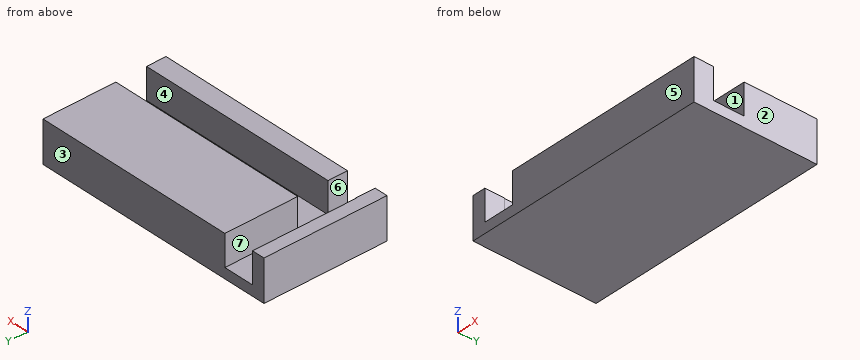
```python
from build123d import *

# Parameters (mm, degrees)
F0_W     = 152.4
F0_H     = 76.2
F1_DEPTH = 25.4
F3_DEPTH = 19.05
F4_W     = 19.05
F4_H     = 19.05
F5_DEPTH = 12.192


with BuildPart() as f1:
    # F0 (on Top) → F1 (new body)
    with BuildSketch(Plane.XY):
        with Locations((24.078096, -6.907338)):
            Rectangle(F0_W, F0_H)
    extrude(amount=F1_DEPTH)

    # F2 (on face) → F3 (cut)
    with BuildSketch(Plane.XY.offset(25.4)):
        Polygon((-25.176978, 31.192662), (-44.226978, 31.192662), (-44.226978, -32.953762), (100.278096, -32.953762), (100.278096, -13.903762), (-25.176978, -13.903762), align=None)
    extrude(amount=-F3_DEPTH, mode=Mode.SUBTRACT)

    # F4 (on face) → F5 (cut)
    with BuildSketch(Plane.XZ.offset(45.007338)):
        with Locations((-34.414173, 15.875)):
            Rectangle(F4_W, F4_H)
    extrude(amount=-F5_DEPTH, mode=Mode.SUBTRACT)


solid = f1.part
```
The listing builds one solid part. Answer for the finished solid, in the listing's coordinates (mm). Face numbers are marked on the shaded views. A direction names the side the tool comes from. Give positions to 0.01 mm unless a question says otherwise; leave off trailing zeros. Order: outer loops, then holes, each group sorted by start corner. A loop starts at its lowest first (then second) coordinate and runs counter-clockwise, first axis right, second up. Notation, with made-up numbers: (9, 20) - (32, 20) arc R15 cw to (32, 38) - close; hole circle Ø8 at (68.25, 29.5). An arc over 180 degrees is marked (long way). Answer in a Markdown table with one row per item. Add a question column.
Q1. The part is cut by section B-B (x = 67). Determine the outline of the cut face in (y, z).
Q2. Which of the six approach directions +Z, -Z, +X, -X, +Y, -Y give full straight-line access (tool end or side, diameter ignored) to the marked faces 5, 6 and 7?
Q3. The part is cut by section A-A (z = 21). Determine the outline of the cut face in (x, y), then the cut area to 3 significant figures.
Q4. The part is cut by section C-C (y = 12.5). Determine the outline of the cut face in (x, z).
Q5. Find the intervals of material crossed by line 1 along X through (y, z) = (-8, 16.5); line 2 along Y through (x, z) = (22.5, 15.75); line 3 along X through (y, z) = (-40.5, 18), in increasing order. Write a range as [from, to].
Q6. For a pull along Y with two mould halves and no side action, classify the marked faces 1, 2, 3 and 4 as released by +Y, released by -Y, zero draft, split by the parting line, or undercut.
Q7. The part is cut by section D-D (y = -30). Determine the outline of the cut face in (x, z).
Determined:
| question | item | result |
|---|---|---|
| 1 | outline | (-45.01, 0) - (31.19, 0) - (31.19, 25.4) - (-13.9, 25.4) - (-13.9, 6.35) - (-32.95, 6.35) - (-32.95, 25.4) - (-45.01, 25.4) - close |
| 2 | face 5 | +Z, -Z, +X, -X, -Y |
| 2 | face 6 | +Z, -Y |
| 2 | face 7 | +Z, +Y, -Y |
| 3 | outline | (-52.12, -45.01) - (-43.94, -45.01) - (-43.94, -32.95) - (-44.23, -32.95) - (-44.23, 31.19) - (-52.12, 31.19) - close; (-25.18, -13.9) - (100.28, -13.9) - (100.28, 31.19) - (-25.18, 31.19) - close; (-24.89, -45.01) - (100.28, -45.01) - (100.28, -32.95) - (-24.89, -32.95) - close |
| 3 | area | 7,770 mm² |
| 4 | outline | (-52.12, 0) - (100.28, 0) - (100.28, 25.4) - (-25.18, 25.4) - (-25.18, 6.35) - (-44.23, 6.35) - (-44.23, 25.4) - (-52.12, 25.4) - close |
| 5 | line 1 | x = [-52.12, -44.23], [-25.18, 100.28] |
| 5 | line 2 | y = [-45.01, -32.95], [-13.9, 31.19] |
| 5 | line 3 | x = [-52.12, -43.94], [-24.89, 100.28] |
| 6 | face 1 | undercut |
| 6 | face 2 | zero draft |
| 6 | face 3 | released by +Y |
| 6 | face 4 | undercut |
| 7 | outline | (-52.12, 0) - (100.28, 0) - (100.28, 6.35) - (-44.23, 6.35) - (-44.23, 25.4) - (-52.12, 25.4) - close |
